```python
from build123d import *

# Parameters (mm, degrees)
SKETCH1_R           = 1.375
SKETCH1_R_2         = 1.460845326
SKETCH1_R_3         = 1.480655282
BOSS_EXTRUDE1_DEPTH = 15
BOSS_EXTRUDE2_START = -8
SKETCH2_R           = 14
SKETCH2_R_2         = 10
BOSS_EXTRUDE2_DEPTH = 8
CUT_EXTRUDE1_START  = -3
SKETCH3_R           = 14
SKETCH3_R_2         = 10
CUT_EXTRUDE1_DEPTH  = 3
SKETCH5_R           = 1.480655282
SKETCH5_R_2         = 1.375
SKETCH5_R_3         = 1.460845326
BOSS_EXTRUDE3_DEPTH = 0.5
BOSS_EXTRUDE4_DEPTH = 5
SKETCH7_R           = 3
CUT_EXTRUDE2_DEPTH  = 12.5
SKETCH8_R           = 14.05
CUT_EXTRUDE3_DEPTH  = 3.5


with BuildPart() as part:
    # Sketch1 → Boss-Extrude1 (new body)
    with BuildSketch(Plane(origin=(0, 0, 0), x_dir=(1, 0, 0), z_dir=(0, 1, 0))):
        with BuildLine():
            Line((-15, -16.85), (15, -16.85))
            Line((15, -16.85), (15, 16.85))
            Line((15, 16.85), (-15, 16.85))
            Line((-15, 16.85), (-15, 2.633913438))
            ThreePointArc((-15, 2.633913438), (0.072875656, 13.937359865), (12.75, 0))
            ThreePointArc((12.75, 0), (0.072875656, -13.937359865), (-15, -2.633913438))
            Line((-15, -2.633913438), (-15, -16.85))
        make_face()
        with Locations(Location((-11.75, -13.5, 0), (0, 0, 270))):
            Circle(SKETCH1_R, mode=Mode.SUBTRACT)
        with Locations(Location((9.25, -13.5, 0), (0, 0, 270))):
            Circle(SKETCH1_R_2, mode=Mode.SUBTRACT)
        with Locations(Location((-11.75, 13.5, 0), (0, 0, 270))):
            Circle(SKETCH1_R, mode=Mode.SUBTRACT)
        with Locations(Location((9.25, 13.5, 0), (0, 0, 270))):
            Circle(SKETCH1_R_3, mode=Mode.SUBTRACT)
    extrude(amount=BOSS_EXTRUDE1_DEPTH)

    # Sketch2 → Boss-Extrude2 (add)
    with BuildSketch(Plane(origin=(0, 15, 0), x_dir=(1, 0, 0), z_dir=(0, 1, 0)).offset(BOSS_EXTRUDE2_START)):
        with Locations((-1.25, 0)):
            Circle(SKETCH2_R)
        with Locations(Location((-1.25, 0, 0), (0, 0, 270))):
            Circle(SKETCH2_R_2, mode=Mode.SUBTRACT)
    extrude(amount=BOSS_EXTRUDE2_DEPTH)

    # Sketch3 → Cut-Extrude1 (cut)
    with BuildSketch(Plane(origin=(0, 15, 0), x_dir=(1, 0, 0), z_dir=(0, 1, 0)).offset(CUT_EXTRUDE1_START)):
        with Locations((-1.25, 0)):
            Circle(SKETCH3_R)
        with Locations(Location((-1.25, 0, 0), (0, 0, 270))):
            Circle(SKETCH3_R_2, mode=Mode.SUBTRACT)
    extrude(amount=CUT_EXTRUDE1_DEPTH, mode=Mode.SUBTRACT)

    # Sketch5 → Boss-Extrude3 (add)
    with BuildSketch(Plane(origin=(0, 15, 0), x_dir=(1, 0, 0), z_dir=(0, 1, 0))):
        with BuildLine():
            Line((-15, 16.85), (-15, 2.633913438))
            ThreePointArc((-15, 2.633913438), (12.75, 0), (-15, -2.633913438))
            Line((-15, -2.633913438), (-15, -16.85))
            Line((-15, -16.85), (15, -16.85))
            Line((15, -16.85), (15, 16.85))
            Line((15, 16.85), (-15, 16.85))
        make_face()
        with Locations(Location((9.25, 13.5, 0), (0, 0, 270))):
            Circle(SKETCH5_R, mode=Mode.SUBTRACT)
        with Locations(Location((-11.75, -13.5, 0), (0, 0, 270))):
            Circle(SKETCH5_R_2, mode=Mode.SUBTRACT)
        with Locations(Location((-11.75, 13.5, 0), (0, 0, 270))):
            Circle(SKETCH5_R_2, mode=Mode.SUBTRACT)
        with Locations(Location((9.25, -13.5, 0), (0, 0, 270))):
            Circle(SKETCH5_R_3, mode=Mode.SUBTRACT)
    extrude(amount=BOSS_EXTRUDE3_DEPTH)

    # Sketch6 → Boss-Extrude4 (add)
    with BuildSketch(Plane(origin=(0, 15.5, 0), x_dir=(1, 0, 0), z_dir=(0, 1, 0))):
        with BuildLine():
            ThreePointArc((-1.625, 20.35), (0, 21.975), (1.625, 20.35))
            Line((1.625, 20.35), (3.5, 20.35))
            ThreePointArc((3.5, 20.35), (0, 23.85), (-3.5, 20.35))
            Line((-3.5, 20.35), (-1.625, 20.35))
        make_face()
        with BuildLine():
            Line((3.5, 20.35), (1.625, 20.35))
            ThreePointArc((1.625, 20.35), (0, 18.725), (-1.625, 20.35))
            Line((-1.625, 20.35), (-3.5, 20.35))
            ThreePointArc((-3.5, 20.35), (-2.474873743, 17.875126275), (-2.6e-08, 16.85))
            ThreePointArc((-2.6e-08, 16.85), (2.474873725, 17.875126257), (3.5, 20.35))
        make_face()
        with BuildLine():
            Line((3.5, 16.85), (3.5, 20.35))
            ThreePointArc((3.5, 20.35), (2.474873725, 17.875126257), (-2.6e-08, 16.85))
            Line((-2.6e-08, 16.85), (3.5, 16.85))
        make_face()
        with BuildLine():
            ThreePointArc((-2.6e-08, 16.85), (-2.474873743, 17.875126275), (-3.5, 20.35))
            Line((-3.5, 20.35), (-3.5, 16.85))
            Line((-3.5, 16.85), (-2.6e-08, 16.85))
        make_face()
        with BuildLine():
            ThreePointArc((-3.5, -20.35), (-2.474873734, -17.875126266), (0, -16.85))
            Line((0, -16.85), (-3.5, -16.85))
            Line((-3.5, -16.85), (-3.5, -20.35))
        make_face()
        with BuildLine():
            Line((3.5, -20.35), (3.5, -16.85))
            Line((3.5, -16.85), (0, -16.85))
            ThreePointArc((0, -16.85), (2.474873734, -17.875126266), (3.5, -20.35))
        make_face()
        with BuildLine():
            ThreePointArc((-3.5, -20.35), (0, -23.85), (3.5, -20.35))
            Line((3.5, -20.35), (1.625, -20.35))
            ThreePointArc((1.625, -20.35), (0, -21.975), (-1.625, -20.35))
            Line((-1.625, -20.35), (-3.5, -20.35))
        make_face()
        with BuildLine():
            Line((1.625, -20.35), (3.5, -20.35))
            ThreePointArc((3.5, -20.35), (2.474873734, -17.875126266), (0, -16.85))
            ThreePointArc((0, -16.85), (-2.474873734, -17.875126266), (-3.5, -20.35))
            Line((-3.5, -20.35), (-1.625, -20.35))
            ThreePointArc((-1.625, -20.35), (0, -18.725), (1.625, -20.35))
        make_face()
    extrude(amount=-BOSS_EXTRUDE4_DEPTH)

    # Sketch7 → Cut-Extrude2 (cut)
    with BuildSketch(Plane(origin=(0, 15.5, 0), x_dir=(1, 0, 0), z_dir=(0, 1, 0))):
        with Locations(Location((-11.75, 13.5, 0), (0, 0, 270))):
            Circle(SKETCH7_R)
        with Locations(Location((9.25, 13.5, 0), (0, 0, 270))):
            Circle(SKETCH7_R)
        with Locations(Location((9.25, -13.5, 0), (0, 0, 270))):
            Circle(SKETCH7_R)
        with Locations(Location((-11.75, -13.5, 0), (0, 0, 270))):
            Circle(SKETCH7_R)
    extrude(amount=-CUT_EXTRUDE2_DEPTH, mode=Mode.SUBTRACT)

    # Sketch8 → Cut-Extrude3 (cut)
    with BuildSketch(Plane(origin=(0, 15.5, 0), x_dir=(1, 0, 0), z_dir=(0, 1, 0))):
        with Locations((-1.25, 0)):
            Circle(SKETCH8_R)
    extrude(amount=-CUT_EXTRUDE3_DEPTH, mode=Mode.SUBTRACT)


solid = part.part
```
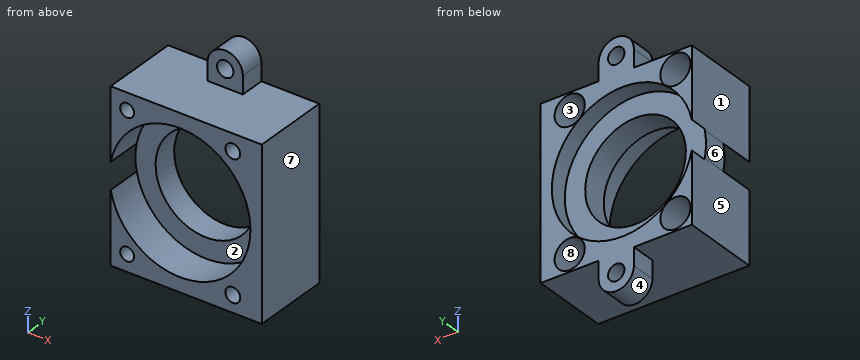
Geometry check sheet. Reference: the model listing, model coordinates, mm. Face numbers are marked on the shaded views. A direction names the side the tool comes from. Round coordinates to 2 decimals unless told otherwise and drop trailing zeros. Order: outer loops, then holes, each group sorted by start corner. A loop starts at its lowest first (then second) coordinate and runs counter-clockwise, first axis right, second up. Notation, with made-up numbers: (15, 69) -> (31, 69) arc R33 cw to (31, 107) -> close; hole circle Ø10 at (34.5, 35.5). An arc over 180 degrees is marked (long way). Return JSON: item names as keys, results as strings. Group by question number.
Q1. Section check C-C, the plane x = -11.75. Record the boundary of the cut face in (y, z) (3 decimals).
Q2. Section check D-D, the plane z = -13. Record the boundary of the cut face in (x, y).
Q3. Gauge pin test, flat ends, axial feed: pin 1 (3 mm diameter, centred on x = -12.5, z = 13.5, fed in from +Y); pin 2 (4 mm diameter, centred on x = 8, y = 6, fed in from -Z); pin 3 (1 mm diameter, centred on y = 10, z = -12.5, fed in from -X); pin 4 (2.5 mm diameter, centred on x = 9.25, z = -13.5, fed in from +Y). Record the tip position at first contact, or that the pin passes through.
Q4. Material ranges on probe 1 along Z at (x, y) = (7, 7.5); probe 2 along Y at (x, z) = (3.5, 9); probe 3 along Z at (x, y) = (9.25, 1.4), recorded low to high. Write a range as from..to.
Q5. Section check A-A, the plane z = -1. Record the boundary of the cut face in (x, y).
Q6. Tool access check on the marked faces 1, 2, 3, 4 and 5. Record the directions out of +Z, -Z, +X, -X, +Y, -Y that give a thin tool (end or side, any length) a straight path to the whole face; none if there is none.
Q7. Section check B-B, the plane y = 6.5. Record the boundary of the cut face in (x, z).
Q8. Release check for a two-part mould opening along X. For the marked faces 6, 7 and 8 record: released by +X, released by -X, zero draft, split by the parting line, or undercut.
Numbers:
{
 "1": {"outline": "(0, -16.85) -> (15.5, -16.85) -> (15.5, -16.5) -> (3, -16.5) -> (3, -14.875) -> (0, -14.875) -> close; (0, -12.125) -> (3, -12.125) -> (3, -10.5) -> (15.5, -10.5) -> (15.5, -9.336) -> (12, -9.336) -> (12, 9.336) -> (15.5, 9.336) -> (15.5, 10.5) -> (3, 10.5) -> (3, 12.125) -> (0, 12.125) -> (0, 9.26) -> (7, 9.26) -> (7, -9.26) -> (0, -9.26) -> close; (0, 14.875) -> (3, 14.875) -> (3, 16.5) -> (15.5, 16.5) -> (15.5, 16.85) -> (0, 16.85) -> close"},
 "2": {"outline": "(-15, 0) -> (-13.03, 0) -> (-13.03, 3) -> (-14.71, 3) -> (-14.71, 15.5) -> (-15, 15.5) -> close; (-10.47, 0) -> (-6.45, 0) -> (-6.45, 7) -> (3.95, 7) -> (3.95, 0) -> (7.86, 0) -> (7.86, 3) -> (6.29, 3) -> (6.29, 15.5) -> (4.08, 15.5) -> (4.08, 12) -> (-6.58, 12) -> (-6.58, 15.5) -> (-8.79, 15.5) -> (-8.79, 3) -> (-10.47, 3) -> close; (10.64, 0) -> (15, 0) -> (15, 15.5) -> (12.21, 15.5) -> (12.21, 3) -> (10.64, 3) -> close"},
 "3": {"pin 1": "y = 3", "pin 2": "z = -16.85", "pin 3": "x = -15", "pin 4": "through"},
 "4": {"probe 1": "-16.85..-15.48, -11.52..-5.65, 5.65..11.52, 15.48..16.85", "probe 2": "7..12", "probe 3": "-16.85..-14.98, -12.02..-9.26, 9.26..12.04, 14.96..16.85"},
 "5": {"outline": "(-15.21, 7) -> (-11.2, 7) -> (-11.2, 12) -> (-15.21, 12) -> close; (8.7, 7) -> (12.71, 7) -> (12.71, 0) -> (15, 0) -> (15, 15.5) -> (12.76, 15.5) -> (12.76, 12) -> (8.7, 12) -> close"},
 "6": {"face 1": "+Z, -X, +Y, -Y", "face 2": "-Y", "face 3": "+Y", "face 4": "-Z, +Y, -Y", "face 5": "-Z, -X, +Y, -Y"},
 "7": {"outline": "(-15, -16.85) -> (15, -16.85) -> (15, 16.85) -> (-15, 16.85) -> (-15, 2.63) arc R14 cw (long way) to (-15, -2.63) -> close; hole circle Ø6 at (-11.75, -13.5); hole circle Ø6 at (-11.75, 13.5); hole circle Ø6 at (9.25, -13.5); hole circle Ø6 at (9.25, 13.5)"},
 "8": {"face 6": "released by -X", "face 7": "released by +X", "face 8": "undercut"}
}
